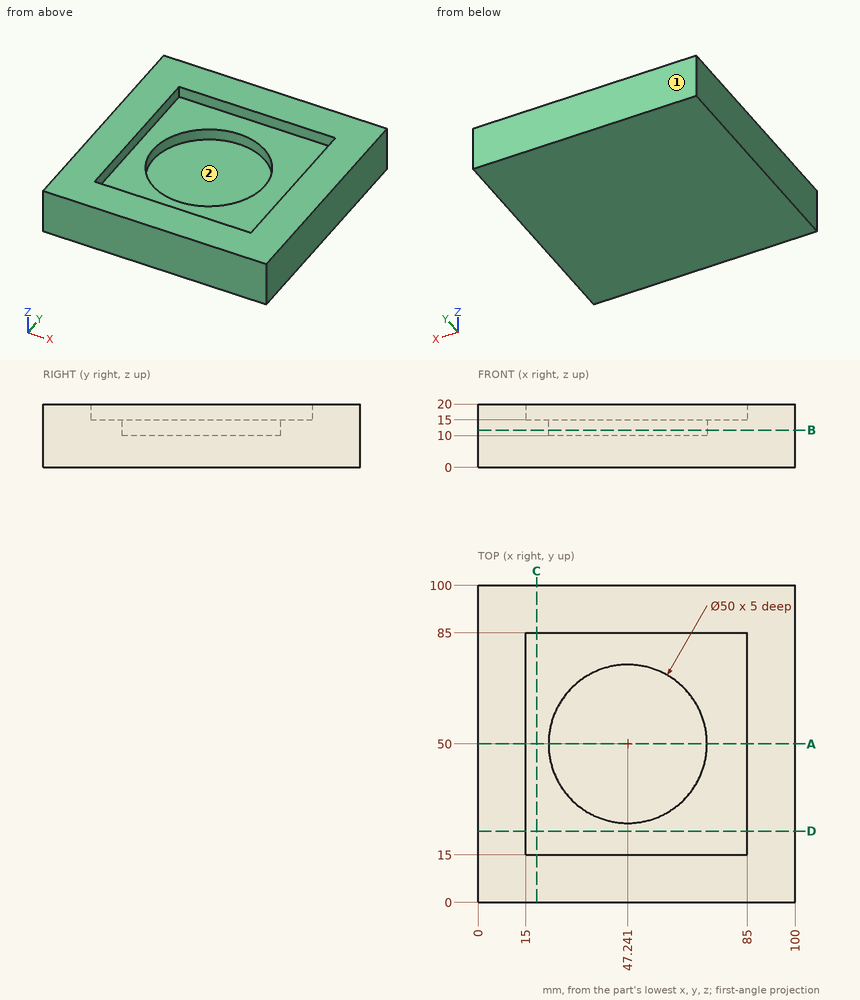
Answer from the drawing. Dimensions are ordinates in mm from the lowest x, y and z of the part. A direction names the side the tool comes from. Give positions to 0.01 mm unless a question says otherwise; leave off trailing zeros. Write each loop counter-clockwise with the first axis right and the second up, starting at its lowest first coordinate (ties: lowest second). Pieces come first, ordered by that corner, then holes. Notation, with made-up numbers: (-5.5, -32.75) - (35.5, -32.75) arc R21 cw to (35.5, -8.75) - close; hole circle Ø1 at (11.25, -26). An arc over 180 degrees is marked (long way). One line per item, written item: value. Start each with the question number.
1. Consider probe 1 along Y at (x, z) = (73.5, 18); probe 2 along X at (y, z) = (49.5, 11); probe 3 along Z at (x, y) = (64, 27). Determine where each line is inside the solid, lowest interval first.
2. Find section B-B (z = 11.75). Write down the section's boundary in (x, y), then the cut area to 3 significant figures.
3. For the marked faces 1 and 2, determine the directions among +Z, -Z, +X, -X, +Y, -Y from which every point of the face is accessible in a straight line to the end or side of a thin tool.
4. Find section C-C (x = 18.5). Write down the section's boundary in (y, z), then the cut area to 3 significant figures.
5. Find section A-A (y = 50). Write down the section's boundary in (x, z), then the cut area to 3 significant figures.
Geometry results:
1. probe 1: 0 to 15, 85 to 100
1. probe 2: 0 to 22.25, 72.24 to 100
1. probe 3: 0 to 15
2. outline: (0, 0) - (100, 0) - (100, 100) - (0, 100) - close; hole circle Ø50 at (47.24, 50)
2. area: 8,040 mm2
3. face 1: +Z, -Z, +X, -X, +Y
3. face 2: +Z
4. outline: (0, 0) - (100, 0) - (100, 20) - (85, 20) - (85, 15) - (15, 15) - (15, 20) - (0, 20) - close
4. area: 1,650 mm2
5. outline: (0, 0) - (100, 0) - (100, 20) - (85, 20) - (85, 15) - (72.24, 15) - (72.24, 10) - (22.24, 10) - (22.24, 15) - (15, 15) - (15, 20) - (0, 20) - close
5. area: 1,400 mm2
